```python
from build123d import *

# Parameters (mm, degrees)
PAD120_DEPTH            = 5
POCKET099_DEPTH         = 3.5
PAD124_DEPTH            = 9
BODY087_PITCH_ANGLE     = 90
BODY087_PLACEMENT_ANGLE = 90


with BuildPart() as part:
    # Sketch244 → Pad120 (new body, symmetric)
    with BuildSketch(Plane.XY):
        with BuildLine():
            Line((-11, 3.7), (-11, -5))
            ThreePointArc((-11, -5), (-10.707107, -5.707107), (-10, -6))
            Line((-10, -6), (10, -6))
            ThreePointArc((10, -6), (10.707107, -5.707107), (11, -5))
            Line((11, -5), (11, 3.7))
            ThreePointArc((11, 3.7), (10.707107, 4.407107), (10, 4.7))
            Line((10, 4.7), (-10, 4.7))
            ThreePointArc((-10, 4.7), (-10.707107, 4.407107), (-11, 3.7))
        make_face()
    extrude(amount=PAD120_DEPTH, both=True)

    # Sketch245 → Pocket099 (cut, symmetric)
    with BuildSketch(Plane.XY):
        Polygon((-10.05, 10), (-10.05, -5), (-9.5, -5), (-9.5, -12), (-7.5, -12), (-7.5, -5), (-2, -5), (-2, -12), (0, -12), (0, -5), (7, -5), (7, -12), (9, -12), (9, -5), (10.05, -5), (10.05, 10), align=None)
    extrude(amount=POCKET099_DEPTH, both=True, mode=Mode.SUBTRACT)

    # Sketch253 (on Face1 of Pocket099) → Pad124 (join)
    with BuildSketch(Plane.YZ.offset(-11)):
        with BuildLine():
            ThreePointArc((-10, -9.25), (-11.75, -11), (-10, -12.75))
            Line((-10, -12.75), (0, -12.75))
            Line((0, -14.75), (0, -12.75))
            Line((-12, -14.75), (0, -14.75))
            ThreePointArc((-14, -12.75), (-13.414214, -14.164214), (-12, -14.75))
            Line((-14, -8.765096), (-14, -12.75))
            ThreePointArc((-12.541491, -6.839794), (-13.594205, -7.557409), (-14, -8.765096))
            Line((-12.541491, -6.839794), (-6, -5))
            Line((0, -5), (-6, -5))
            Line((0, -9.25), (0, -5))
            Line((-10, -9.25), (0, -9.25))
        make_face()
    pad124 = extrude(amount=PAD124_DEPTH)

    # Mirrored012: Pad124 across Sketch253 V_Axis
    add(pad124.mirror(Plane(origin=(-11, 0, 0), x_dir=(1, 0, 0), z_dir=(0, 1, 0))))


with BuildPart() as part_1:
    # Body087 pitch: moved
    add(part.part.rotate(Axis((0, 0, 0), (0, 1, 0)), BODY087_PITCH_ANGLE))


with BuildPart() as part_2:
    # Body087 placement: moved
    add(part_1.part.moved(Location((0, 0, 0))).rotate(Axis((0, 0, 0), (0, 0, 1)), BODY087_PLACEMENT_ANGLE))


solid = part_2.part
```
The model under review builds one solid part; all positions refer to its coordinate system, in mm. A direction names the side the tool comes from. Round coordinates to 2 decimals unless told otherwise and drop trailing zeros. Write each loop counter-clockwise with the first axis right and the second up, starting at its lowest first coordinate (ties: lowest second). Pieces come first, ordered by that corner, then holes. Notation, with made-up numbers: M 72,4.25 L 118,4.25 A17 cw 118,28.25 Z; hole C -39,28 d5. An arc over 180 degrees is marked long. Use CSV: the item, a comma, the result in double quotes. Start each with the question number.
(1) We need section C-C, the plane z = -8. State the section outline as (x, y) points.
(2) For line 1 along Y through (x, z) = (0.5, 6.5); line 2 along Y through (x, z) = (5.5, 0.75); line 3 along Z through (x, y) = (-2.25, 0.75), list the stretches that pass through material, from the lowest coordinate up.
(3) We need section B-B, the plane y = -11. State the section outline as (x, z) points.
(4) We need section D-D, the plane y = 2. State the section outline as (x, z) points, then the cut area to 3 significant figures.
(5) Tool access review of faces 4 (the face through (1, 3.5, 0)), 5 (the face through (6, 0, -2)), 6 (the face through (5.5, 0, 2)): name each direction out of +Z, -Z, +X, -X, +Y, -Y from which nothing blocks a thin tool from reaching the whole face with its end or side.
(6) The part is to be moulded in two halves that separate along Y. For faces 1 (the face through (0, 0, -10.05)), 2 (the face through (14, -11, 7)), 3 (the face through (1, -5, -4)), say which applies: +Y half, -Y half, draft (parallel to the pull), parting line (faces both ways), or undercut.
(7) Clearance check with flat-ended pins moving along their axes: P1, Ø1.7, axis at y = -4, z = -3, coming from the -X side; P2, Ø5.5, axis at x = 0.5, z = -3, coming from the -Y side; P3, Ø0.5, axis at x = 5.5, y = -0.5, coming from the +Z side; P4, Ø3, axis at x = -2, y = -11, coming from the -Z side. State where each tip first meets the part, or that it passes through.
(8) We need section A-A, the plane x = -2.75. State the section outline as (y, z) points, then the cut area to 3 significant figures.
Findings:
1,outline,"M -4.7,-5 L 6,-5 L 6,-3.5 L -4.7,-3.5 Z; M -4.7,3.5 L 6,3.5 L 6,5 L -4.7,5 Z"
2,line 1,"-14.75 to -12.75, -9.25 to -3.5, 3.5 to 5"
2,line 2,"-5 to -3.5, 3.5 to 5"
2,line 3,"-11 to -10.05, 10.05 to 11"
3,outline,"M -14,2 L -11.75,2 L -11.75,11 L -14,11 Z; M 11.75,2 L 14,2 L 14,11 L 11.75,11 Z"
4,outline,"M -4.7,-10.05 A1 ccw -3.7,-11 L 5,-11 A1 ccw 6,-10 L 6,-9 L 5,-9 L 5,-10.05 Z; M -4.7,10.05 L 5,10.05 L 5,9.5 L 6,9.5 L 6,10 A1 ccw 5,11 L -3.7,11 A1 ccw Z; M 5,-7 L 6,-7 L 6,0 L 5,0 Z; M 5,2 L 6,2 L 6,7.5 L 5,7.5 Z"
4,area,"33.6 mm^2"
5,face 4,"-X"
5,face 5,"+Z, -Z, +X, +Y"
5,face 6,"+X, -X"
6,face 1,"undercut"
6,face 2,"draft"
6,face 3,"-Y half"
7,P1,"x = -4.7"
7,P2,"y = -5"
7,P3,"z = 10.97"
7,P4,"through"
8,outline,"M -14.75,2 L -12.75,2 L -12.75,11 L -14.75,11 Z; M -9.25,2 L -5,2 L -5,-11 L 5,-11 L 5,11 L -9.25,11 Z; hole M -3.5,-10.05 L 3.5,-10.05 L 3.5,10.05 L -3.5,10.05 Z"
8,area,"136 mm^2"
